For this review, take the finished solid that the model builds, in its own axes (mm). A direction names the side the tool comes from. Round coordinates to 2 decimals unless told otherwise and drop trailing zeros. Order: outer loops, then holes, each group sorted by start corner. A loop starts at its lowest first (then second) coordinate and runs counter-clockwise, first axis right, second up. Notation, with made-up numbers: (62.25, 81.5) -> (113.25, 81.5) arc R18 ccw to (113.25, 88.5) -> close; hole circle Ø8 at (51.5, -6). An arc over 180 degrees is marked (long way). Use a Markdown table: item, result. Add a question column.
1) Wall thickness on line 1 along Z through (x, y) = (13.5, 14); line 2 along Z through (x, y) = (-0.25, 12); line 3 along X through (y, z) = (5.25, 13): over which ranges is each line inside the solid? List them lowest first. Write a range as [from, to].
2) Consider section C-C (x = -2). State the section outline as (y, z) points, plus the area to 3 significant figures.
3) Clearance check with flat-ended pins moving along their axes: P1, Ø2, axis at x = 6.5, y = -3, coming from the +Z side; P2, Ø4.5, axis at x = -3, y = -4.5, coming from the -Z side; P3, Ø2, axis at x = 10.5, z = 16, coming from the -Y side. State where each tip first meets the part, or that it passes through.
4) Consider section B-B (z = 10). State the section outline as (x, y) points.
5) Consider section A-A (z = -7). State the section outline as (x, y) points (3 decimals).
6) Draft analysis for pull direction Z (two halves, no side actions). For faces 5 (the face through (1, -3, 19)), 6 (the face through (0, 9, -20)), 7 (the face through (-14.55, 9.61, 29.57)), state which applies: pulls with the +Z half, pulls with the -Z half, needs draft (parallel to the pull), parting line crosses it, or undercut.
7) Machinability: for faces 1 (the face through (-7, -3, 17)), 2 (the face through (-13.4, 16.5, 12.4)), 3 (the face through (14, 13, 23)), 4 (the face through (-14, 12, -7)), which of the approach directions +Z, -Z, +X, -X, +Y, -Y give a long, thin tool a straight path to every point of the face, cutting with its end or side? Answer none if there is none.
```python
from build123d import *

# Parameters (mm, degrees)
BOSS_EXTRUDE1_DEPTH = 17.5
SHELL1_T            = -2
FILLET1_R           = 1.5
CUT_EXTRUDE3_REACH  = 4
SKETCH7_W           = 11
SKETCH7_H           = 2.5
CUT_EXTRUDE4_REACH  = 4
SKETCH8_W           = 11
SKETCH8_H           = 2.5
CUT_EXTRUDE5_DEPTH  = 1
CUT_EXTRUDE6_REACH  = 52
BOSS_EXTRUDE2_DEPTH = 6
FILLET2_R           = 2
FILLET3_R           = 1


with BuildPart() as part:
    # Sketch1 → Boss-Extrude1 (new body)
    with BuildSketch(Plane(origin=(0, 0, 0), x_dir=(1, 0, 0), z_dir=(0, 1, 0))):
        Polygon((-15, 20), (15, 20), (15, -20), (15, -30), (-15, -30), (-15, -20), align=None)
    extrude(amount=BOSS_EXTRUDE1_DEPTH)

    # Shell1
    shell1_openings = [part.faces().sort_by_distance(p)[0] for p in [
        (0, 17.5, 5),
    ]]
    offset(amount=SHELL1_T, openings=shell1_openings, kind=Kind.INTERSECTION)

    # Fillet1
    fillet1_edges = [part.edges().sort_by_distance(p)[0] for p in [
        (15, 8.75, 30),
        (-15, 8.75, 30),
        (-15, 8.75, -20),
        (15, 8.75, -20),
        (0, 0, 30),
        (-15, 0, 5),
        (0, 0, -20),
        (15, 0, 5),
    ]]
    fillet(fillet1_edges, radius=FILLET1_R)

    # Sketch7 → Cut-Extrude3 (cut, up to next)
    with BuildSketch(Plane.ZY.offset(-13), mode=Mode.PRIVATE) as cut_extrude3_sk1:
        with Locations((17.5, 13.25)):
            Rectangle(SKETCH7_W, SKETCH7_H)
    cut_extrude3_tool1 = extrude(cut_extrude3_sk1.sketch, amount=-CUT_EXTRUDE3_REACH, mode=Mode.PRIVATE) & part.part
    add(cut_extrude3_tool1.solids().sort_by_distance((13, 13.25, 17.5))[0], mode=Mode.SUBTRACT)

    # Sketch8 → Cut-Extrude4 (cut, up to next)
    with BuildSketch(Plane(origin=(-13, 0, 0), x_dir=(0, 0, -1), z_dir=(1, 0, 0)), mode=Mode.PRIVATE) as cut_extrude4_sk1:
        with Locations((7.5, 13.25)):
            Rectangle(SKETCH8_W, SKETCH8_H)
    cut_extrude4_tool1 = extrude(cut_extrude4_sk1.sketch, amount=-CUT_EXTRUDE4_REACH, mode=Mode.PRIVATE) & part.part
    add(cut_extrude4_tool1.solids().sort_by_distance((-13, 13.25, -7.5))[0], mode=Mode.SUBTRACT)

    # Sketch9 → Cut-Extrude5 (cut)
    with BuildSketch(Plane(origin=(0, 17.5, 0), x_dir=(1, 0, 0), z_dir=(0, 1, 0))):
        Polygon((-13, 18), (-14, 18), (-14, -19), (-14, -29), (14, -29), (14, -19), (14, 18), (13, 18), (13, -18), (13, -28), (-13, -28), (-13, -18), align=None)
    extrude(amount=-CUT_EXTRUDE5_DEPTH, mode=Mode.SUBTRACT)

    # Sketch10 → Cut-Extrude6 (cut, up to next)
    with BuildSketch(Plane.XY.offset(30), mode=Mode.PRIVATE) as cut_extrude6_sk1:
        with BuildLine():
            Line((-3, 17.5), (3, 17.5))
            ThreePointArc((3, 17.5), (0, 14.5), (-3, 17.5))
        make_face()
    cut_extrude6_tool1 = extrude(cut_extrude6_sk1.sketch, amount=-CUT_EXTRUDE6_REACH, mode=Mode.PRIVATE) & part.part
    add(cut_extrude6_tool1.solids().sort_by_distance((0, 16.22676, 30))[0], mode=Mode.SUBTRACT)

    # Sketch11 → Boss-Extrude2 (add)
    with BuildSketch(Plane.XZ):
        Polygon((-9, 21.5), (-9, -11.5), (6.25, -11.5), (9, -11.5), (9, 21.5), (7, 21.5), align=None)
        Polygon((-7, 5.524400968), (0, 5.524400968), (0, 8.324400968), (1, 8.324400968), (1, 5.524400968), (7, 5.524400968), (7, 12.524400968), (5.2, 12.524400968), (5.2, 13.524400968), (7, 13.524400968), (7, 19.524400968), (6.25, 19.524400968), (1, 19.524400968), (1, 17.724400968), (0, 17.724400968), (0, 19.524400968), (-7, 19.524400968), (-7, 13.524400968), (-4.2, 13.524400968), (-4.2, 12.524400968), (-7, 12.524400968), align=None, mode=Mode.SUBTRACT)
        Polygon((7.285005864, -9.5), (6.535005864, -9.5), (1.285005864, -9.5), (1.285005864, -7.7), (0.285005864, -7.7), (0.285005864, -9.5), (-6.714994136, -9.5), (-7, -9.5), (-7, -3.5), (-6.714994136, -3.5), (-3.914994136, -3.5), (-3.914994136, -2.475599032), (-7, -2.475599032), (-7, 4.524400968), (0, 4.524400968), (0, 1.724400968), (1, 1.724400968), (1, 4.524400968), (7.285005864, 4.524400968), (7.285005864, -2.5), (5.485005864, -2.5), (5.485005864, -3.5), (7.285005864, -3.5), align=None, mode=Mode.SUBTRACT)
    extrude(amount=BOSS_EXTRUDE2_DEPTH)

    # Fillet2
    fillet2_edges = [part.edges().sort_by_distance(p)[0] for p in [
        (-9, 0, 5),
        (0, 0, -11.5),
        (0, 0, 21.5),
        (9, 0, 5),
    ]]
    fillet(fillet2_edges, radius=FILLET2_R)

    # Fillet3
    fillet3_edges = [part.edges().sort_by_distance(p)[0] for p in [
        (0.785005864, -6, -7.7),
        (5.2, -6, 13.024400968),
        (0.5, -6, 8.324400968),
        (-4.2, -6, 13.024400968),
        (0.5, -6, 17.724400968),
        (-3.914994136, -6, -2.987799516),
        (0.5, -6, 1.724400968),
        (5.485005864, -6, -3),
    ]]
    fillet(fillet3_edges, radius=FILLET3_R)


solid = part.part
```
Results list:
| question | item | result |
|---|---|---|
| 1 | line 1 | [-20, 12], [23, 30] |
| 1 | line 2 | [-20, -18], [28, 30] |
| 1 | line 3 | [-15, -13], [13, 15] |
| 2 | outline | (-6, -11.5) -> (-2, -11.5) arc R2 cw to (0, -13.5) -> (0, -18.5) arc R1.5 ccw to (1.5, -20) -> (17.5, -20) -> (17.5, -18) -> (2, -18) -> (2, 28) -> (15.26, 28) -> (15.26, 30) -> (1.5, 30) arc R1.5 ccw to (0, 28.5) -> (0, 23.5) arc R2 cw to (-2, 21.5) -> (-6, 21.5) -> (-6, 19.52) -> (0, 19.52) -> (0, 5.52) -> (-6, 5.52) -> (-6, 4.52) -> (0, 4.52) -> (0, -9.5) -> (-6, -9.5) -> close |
| 2 | area | 188 mm2 |
| 3 | P1 | z = 21.5 |
| 3 | P2 | z = -11.5 |
| 3 | P3 | y = -0.68 |
| 4 | outline | (-15, 1.5) arc R1.5 ccw to (-13.5, 0) -> (-11, 0) arc R2 cw to (-9, -2) -> (-9, -6) -> (-7, -6) -> (-7, 0) -> (7, 0) -> (7, -6) -> (9, -6) -> (9, -2) arc R2 cw to (11, 0) -> (13.5, 0) arc R1.5 ccw to (15, 1.5) -> (15, 17.5) -> (14, 17.5) -> (14, 16.5) -> (13, 16.5) -> (13, 2) -> (-13, 2) -> (-13, 16.5) -> (-14, 16.5) -> (-14, 17.5) -> (-15, 17.5) -> close |
| 5 | outline | (-15, 1.5) arc R1.5 ccw to (-13.5, 0) -> (-11, 0) arc R2 cw to (-9, -2) -> (-9, -6) -> (-7, -6) -> (-7, 0) -> (7.285, 0) -> (7.285, -6) -> (9, -6) -> (9, -2) arc R2 cw to (11, 0) -> (13.5, 0) arc R1.5 ccw to (15, 1.5) -> (15, 17.5) -> (14, 17.5) -> (14, 16.5) -> (13, 16.5) -> (13, 2) -> (-13, 2) -> (-13, 12) -> (-15, 12) -> close; (-15, 14.5) -> (-13, 14.5) -> (-13, 16.5) -> (-14, 16.5) -> (-14, 17.5) -> (-15, 17.5) -> close |
| 6 | face 5 | undercut |
| 6 | face 6 | pulls with the -Z half |
| 6 | face 7 | pulls with the +Z half |
| 7 | face 1 | -Y |
| 7 | face 2 | +Y |
| 7 | face 3 | +X |
| 7 | face 4 | -X |
